from build123d import *

# Parameters (mm, degrees)
SKETCH1_R           = 95
BOSS_EXTRUDE1_DEPTH = 16
SKETCH2_R           = 35
CUT_EXTRUDE1_DEPTH  = 136.299667405
SKETCH3_R           = 10
CUT_EXTRUDE2_DEPTH  = 13.369874
CIRPATTERN1_START   = 2.630125735
CIRPATTERN1_DEPTH   = 13.369874265


# Read off the part's stored shape, not the designer's step: CirPattern1
with BuildPart() as part:
    # Sketch1 → Boss-Extrude1 (new body)
    with BuildSketch(Plane(origin=(0, 0, 0), x_dir=(1, 0, 0), z_dir=(0, 1, 0))):
        with Locations(Location((0, 0, 0), (0, 0, 270))):
            Circle(SKETCH1_R)
    extrude(amount=BOSS_EXTRUDE1_DEPTH)

    # Sketch2 → Cut-Extrude1 (cut, through all)
    with BuildSketch(Plane(origin=(0, 0, 0), x_dir=(1, 0, 0), z_dir=(0, 1, 0))):
        with Locations(Location((0, 0, 0), (0, 0, 270))):
            Circle(SKETCH2_R)
    extrude(amount=CUT_EXTRUDE1_DEPTH, mode=Mode.SUBTRACT)

    # Sketch3 → Cut-Extrude2 (cut)
    with BuildSketch(Plane(origin=(0, 16, 0), x_dir=(1, 0, 0), z_dir=(0, 1, 0))):
        with Locations((-31.056865323, 0)):
            Circle(SKETCH3_R)
    extrude(amount=-CUT_EXTRUDE2_DEPTH, mode=Mode.SUBTRACT)

    # CirPattern1 outline → CirPattern1 (cut)
    with BuildSketch(Plane(origin=(0, 0, 0), x_dir=(1, 0, 0), z_dir=(0, 1, 0)).offset(CIRPATTERN1_START)):
        with BuildLine():
            ThreePointArc((-16.956319822, -30.618347736), (-24.748737342, -24.748737342), (-30.618347736, -16.956319822))
            ThreePointArc((-30.618347736, -16.956319822), (-29.031587884, -29.031587884), (-16.956319822, -30.618347736))
        make_face()
        with BuildLine():
            ThreePointArc((-16.956319822, 30.618347736), (-29.031587884, 29.031587884), (-30.618347736, 16.956319822))
            ThreePointArc((-30.618347736, 16.956319822), (-24.748737342, 24.748737342), (-16.956319822, 30.618347736))
        make_face()
        with BuildLine():
            ThreePointArc((9.660512583, -33.640370043), (0, -35), (-9.660512583, -33.640370043))
            ThreePointArc((-9.660512583, -33.640370043), (0, -41.056865323), (9.660512583, -33.640370043))
        make_face()
        with BuildLine():
            ThreePointArc((9.660512583, 33.640370043), (0, 41.056865323), (-9.660512583, 33.640370043))
            ThreePointArc((-9.660512583, 33.640370043), (0, 35), (9.660512583, 33.640370043))
        make_face()
        with BuildLine():
            ThreePointArc((30.618347736, -16.956319822), (24.748737342, -24.748737342), (16.956319822, -30.618347736))
            ThreePointArc((16.956319822, -30.618347736), (29.031587884, -29.031587884), (30.618347736, -16.956319822))
        make_face()
        with BuildLine():
            ThreePointArc((30.618347736, 16.956319822), (29.031587884, 29.031587884), (16.956319822, 30.618347736))
            ThreePointArc((16.956319822, 30.618347736), (24.748737342, 24.748737342), (30.618347736, 16.956319822))
        make_face()
        with BuildLine():
            ThreePointArc((33.640370043, 9.660512583), (35, 0), (33.640370043, -9.660512583))
            ThreePointArc((33.640370043, -9.660512583), (41.056865323, 0), (33.640370043, 9.660512583))
        make_face()
    extrude(amount=CIRPATTERN1_DEPTH, mode=Mode.SUBTRACT)


solid = part.part
Work out the finished part from the listing and answer in its coordinate system (mm). A direction names the side the tool comes from. Round coordinates to 2 decimals unless told otherwise and drop trailing zeros. Loops run counter-clockwise (first coordinate to the right, second up) from the corner with the lowest first, then second, coordinate; pieces in that order, holes last. Notation, with made-up numbers: M 87,13 L 128,13 A28 ccw 128,43 Z; hole C -22,-35 d7. An arc over 180 degrees is marked long. One line per question, with ' | ' between items. Start each with the question number.
(1) A cutting plane is placed at B-B on x = 0. Write down the section's boundary in (y, z), plus the area to 3 significant figures.
(2) Flat-ended cylindrical pins translate along their axes: pin 1 Ø16.5 at (x, z) = (-21.5, -23) entering from +Y; pin 2 Ø8 at (y, z) = (9.5, -14) entering from -X; pin 3 Ø1.5 at (x, y) = (-32.5, 2.5) entering from +Z. Find the tip coordinate at first contact, or state that the pin passes through.
(3) Find the intervals of material crossed by line 1 (X direction, y = 9.5, z = 0); line 2 (Z direction, x = -7.5, y = 10.25); line 3 (X direction, y = 4.25, z = 19), in increasing order.
(4) A tool of negligible diameter and unlimited length cuts with its end or side. For faces 4 (the face through (41.055, 9.221, 0.183)), 5 (the face through (1, 0, 41)), from which of +Z, -Z, +X, -X, +Y, -Y can it reach the whole face along a straight path? Write none if from no direction.
(5) A cutting plane is placed at D-D on x = -74. Write down the section's boundary in (y, z), plus the area to 3 significant figures.
(6) A cutting plane is placed at C-C on y = 13.25. Write down the section's boundary in (x, z).
(7) For a pull along Z with two mould halves and no side action, classify faces 1 (the face through (-92.74, 7.89, -20.59)), 2 (the face through (0.183, 9.221, -41.055)), 3 (the face through (-20, 16, 41)) as released by +Z, released by -Z, zero draft, split by the parting line, or undercut.
(8) A cutting plane is placed at A-A on z = 0. Write down the section's boundary in (x, y), plus the area to 3 significant figures.
Geometry check:
1) outline: M 0,-95 L 16,-95 L 16,-41.06 L 2.63,-41.06 L 2.63,-35 L 0,-35 Z; M 0,35 L 2.63,35 L 2.63,41.06 L 16,41.06 L 16,95 L 0,95 Z | area: 1,760 mm²
2) pin 1: stops at y = 2.63 | pin 2: stops at x = -94.47 | pin 3: stops at z = 89.54
3) line 1: x = -95 to -41.06, 41.06 to 95 | line 2: z = -94.7 to -37.67, 37.67 to 94.7 | line 3: x = -93.08 to -31.51, 31.51 to 93.08
4) face 4: +Y | face 5: +Z, -Z, +X, -X, -Y
5) outline: M 0,-59.57 L 16,-59.57 L 16,59.57 L 0,59.57 Z | area: 1,910 mm²
6) outline: C 0,0 d190; hole M -33.64,-9.66 A35 ccw -30.62,-16.96 A10 ccw -16.96,-30.62 A35 ccw -9.66,-33.64 A10 ccw 9.66,-33.64 A35 ccw 16.96,-30.62 A10 ccw 30.62,-16.96 A35 ccw 33.64,-9.66 A10 ccw 33.64,9.66 A35 ccw 30.62,16.96 A10 ccw 16.96,30.62 A35 ccw 9.66,33.64 A10 ccw -9.66,33.64 A35 ccw -16.96,30.62 A10 ccw -30.62,16.96 A35 ccw -33.64,9.66 A10 ccw Z
7) face 1: split by the parting line | face 2: undercut | face 3: zero draft
8) outline: M -95,0 L -35,0 L -35,2.63 L -41.06,2.63 L -41.06,16 L -95,16 Z; M 35,0 L 95,0 L 95,16 L 41.06,16 L 41.06,2.63 L 35,2.63 Z | area: 1,760 mm²
